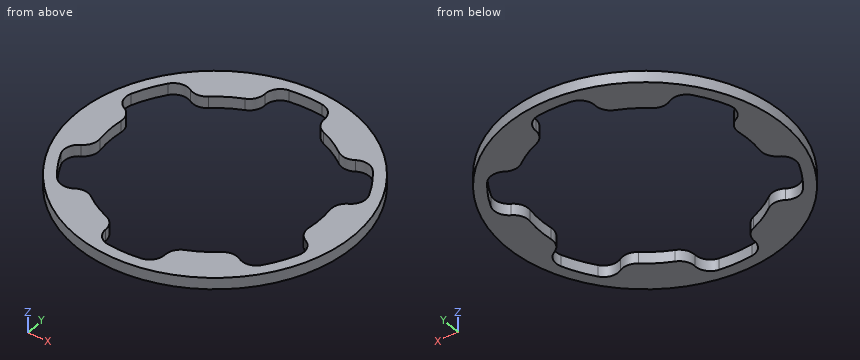
Autodesk Inventor part; units mm, degrees
ref_plane "YZ Plane" through (0, 0, 0) normal (1, 0, 0) x (0, 1, 0)
ref_plane "XZ Plane" through (0, 0, 0) normal (0, 1, 0) x (-1, 0, 0)
ref_plane "XY Plane" through (0, 0, 0) normal (0, 0, 1) x (1, 0, 0)
sketch "MAXSpline Spacer Profile" plane through (0, 0, 0) normal (0, 0, 1) x (1, 0, 0)
  circle A0 centre (0, 0) radius 19.05
  arc A1 (15.22, 4.1356) -> (16.1399, 6.7328) centre (14.2452, 5.9424) ccw
  arc A2 (15.22, 4.1356) -> (14.1626, 2.0366) centre (16.1947, 2.3288) ccw
  arc A3 (14.1626, -2.0366) -> (14.1626, 2.0366) centre (0, 0) ccw
  arc A4 (14.1626, -2.0366) -> (15.22, -4.1356) centre (16.1947, -2.3288) ccw
  arc A5 (16.1399, -6.7328) -> (15.22, -4.1356) centre (14.2452, -5.9424) ccw
  arc A6 (13.9007, -10.6112) -> (16.1399, -6.7328) centre (0, 0) ccw
  arc A7 (11.1915, -11.1131) -> (13.9007, -10.6112) centre (12.2689, -9.3655) ccw
  arc A8 (11.1915, -11.1131) -> (8.845, -11.2469) centre (10.1141, -12.8607) ccw
  arc A9 (5.3176, -13.2835) -> (8.845, -11.2469) centre (0, 0) ccw
  arc A10 (5.3176, -13.2835) -> (4.0285, -15.2487) centre (6.0806, -15.1894) ccw
  arc A11 (2.2392, -17.344) -> (4.0285, -15.2487) centre (1.9763, -15.3079) ccw
  arc A12 (-2.2392, -17.344) -> (2.2392, -17.344) centre (0, 0) ccw
  arc A13 (-4.0285, -15.2487) -> (-2.2392, -17.344) centre (-1.9763, -15.3079) ccw
  arc A14 (-4.0285, -15.2487) -> (-5.3176, -13.2835) centre (-6.0806, -15.1894) ccw
  arc A15 (-8.845, -11.2469) -> (-5.3176, -13.2835) centre (0, 0) ccw
  arc A16 (-8.845, -11.2469) -> (-11.1915, -11.1131) centre (-10.1141, -12.8607) ccw
  arc A17 (-13.9007, -10.6112) -> (-11.1915, -11.1131) centre (-12.2689, -9.3655) ccw
  arc A18 (-16.1399, -6.7328) -> (-13.9007, -10.6112) centre (0, 0) ccw
  arc A19 (-15.22, -4.1356) -> (-16.1399, -6.7328) centre (-14.2452, -5.9424) ccw
  arc A20 (-15.22, -4.1356) -> (-14.1626, -2.0366) centre (-16.1947, -2.3288) ccw
  arc A21 (-14.1626, 2.0366) -> (-14.1626, -2.0366) centre (0, 0) ccw
  arc A22 (-14.1626, 2.0366) -> (-15.22, 4.1356) centre (-16.1947, 2.3288) ccw
  arc A23 (-16.1399, 6.7328) -> (-15.22, 4.1356) centre (-14.2452, 5.9424) ccw
  arc A24 (-13.9007, 10.6112) -> (-16.1399, 6.7328) centre (0, 0) ccw
  arc A25 (-11.1915, 11.1131) -> (-13.9007, 10.6112) centre (-12.2689, 9.3655) ccw
  arc A26 (-11.1915, 11.1131) -> (-8.845, 11.2469) centre (-10.1141, 12.8607) ccw
  arc A27 (-5.3176, 13.2835) -> (-8.845, 11.2469) centre (0, 0) ccw
  arc A28 (-5.3176, 13.2835) -> (-4.0285, 15.2487) centre (-6.0806, 15.1894) ccw
  arc A29 (-2.2392, 17.344) -> (-4.0285, 15.2487) centre (-1.9763, 15.3079) ccw
  arc A30 (2.2392, 17.344) -> (-2.2392, 17.344) centre (0, 0) ccw
  arc A31 (4.0285, 15.2487) -> (2.2392, 17.344) centre (1.9763, 15.3079) ccw
  arc A32 (4.0285, 15.2487) -> (5.3176, 13.2835) centre (6.0806, 15.1894) ccw
  arc A33 (8.845, 11.2469) -> (5.3176, 13.2835) centre (0, 0) ccw
  arc A34 (8.845, 11.2469) -> (11.1915, 11.1131) centre (10.1141, 12.8607) ccw
  arc A35 (13.9007, 10.6112) -> (11.1915, 11.1131) centre (12.2689, 9.3655) ccw
  arc A36 (16.1399, 6.7328) -> (13.9007, 10.6112) centre (0, 0) ccw
  arc A37 (17.4067, -2.0716) -> (17.4067, 2.0716) centre (0, 0) ccw
  arc A38 (15.7454, -1.8738) -> (17.4067, -2.0716) centre (16.5761, -1.9727) ccw
  arc A39 (15.7454, -1.8738) -> (15.7454, 1.8738) centre (0, 0) ccw
  arc A40 (17.4067, 2.0716) -> (15.7454, 1.8738) centre (16.5761, 1.9727) ccw
  arc A41 (10.4974, 14.0389) -> (6.9093, 16.1104) centre (0, 0) ccw
  arc A42 (9.4955, 12.699) -> (10.4974, 14.0389) centre (9.9964, 13.3689) ccw
  arc A43 (9.4955, 12.699) -> (6.2499, 14.5728) centre (0, 0) ccw
  arc A44 (6.9093, 16.1104) -> (6.2499, 14.5728) centre (6.5796, 15.3416) ccw
  arc A45 (-6.9093, 16.1104) -> (-10.4974, 14.0389) centre (0, 0) ccw
  arc A46 (-6.2499, 14.5728) -> (-6.9093, 16.1104) centre (-6.5796, 15.3416) ccw
  arc A47 (-6.2499, 14.5728) -> (-9.4955, 12.699) centre (0, 0) ccw
  arc A48 (-10.4974, 14.0389) -> (-9.4955, 12.699) centre (-9.9964, 13.3689) ccw
  arc A49 (-17.4067, 2.0716) -> (-17.4067, -2.0716) centre (0, 0) ccw
  arc A50 (-15.7454, 1.8738) -> (-17.4067, 2.0716) centre (-16.5761, 1.9727) ccw
  arc A51 (-15.7454, 1.8738) -> (-15.7454, -1.8738) centre (0, 0) ccw
  arc A52 (-17.4067, -2.0716) -> (-15.7454, -1.8738) centre (-16.5761, -1.9727) ccw
  arc A53 (-10.4974, -14.0389) -> (-6.9093, -16.1104) centre (0, 0) ccw
  arc A54 (-9.4955, -12.699) -> (-10.4974, -14.0389) centre (-9.9964, -13.3689) ccw
  arc A55 (-9.4955, -12.699) -> (-6.2499, -14.5728) centre (0, 0) ccw
  arc A56 (-6.9093, -16.1104) -> (-6.2499, -14.5728) centre (-6.5796, -15.3416) ccw
  arc A57 (6.9093, -16.1104) -> (10.4974, -14.0389) centre (0, 0) ccw
  arc A58 (6.2499, -14.5728) -> (6.9093, -16.1104) centre (6.5796, -15.3416) ccw
  arc A59 (6.2499, -14.5728) -> (9.4955, -12.699) centre (0, 0) ccw
  arc A60 (10.4974, -14.0389) -> (9.4955, -12.699) centre (9.9964, -13.3689) ccw
  dimension "d0" = 38.1
sketch "Sketch1" plane through (0, 0, 0) normal (0, 0, 1) x (1, 0, 0)
  circle A0 centre (0, 0) radius 19.05
  arc A1 (15.22, 4.1356) -> (16.1399, 6.7328) centre (14.2452, 5.9424) ccw
  arc A2 (15.22, 4.1356) -> (14.1626, 2.0366) centre (16.1947, 2.3288) ccw
  arc A3 (14.1626, -2.0366) -> (14.1626, 2.0366) centre (0, 0) ccw
  arc A4 (14.1626, -2.0366) -> (15.22, -4.1356) centre (16.1947, -2.3288) ccw
  arc A5 (16.1399, -6.7328) -> (15.22, -4.1356) centre (14.2452, -5.9424) ccw
  arc A6 (13.9007, -10.6112) -> (16.1399, -6.7328) centre (0, 0) ccw
  arc A7 (11.1915, -11.1131) -> (13.9007, -10.6112) centre (12.2689, -9.3655) ccw
  arc A8 (11.1915, -11.1131) -> (8.845, -11.2469) centre (10.1141, -12.8607) ccw
  arc A9 (5.3176, -13.2835) -> (8.845, -11.2469) centre (0, 0) ccw
  arc A10 (5.3176, -13.2835) -> (4.0285, -15.2487) centre (6.0806, -15.1894) ccw
  arc A11 (2.2392, -17.344) -> (4.0285, -15.2487) centre (1.9763, -15.3079) ccw
  arc A12 (-2.2392, -17.344) -> (2.2392, -17.344) centre (0, 0) ccw
  arc A13 (-4.0285, -15.2487) -> (-2.2392, -17.344) centre (-1.9763, -15.3079) ccw
  arc A14 (-4.0285, -15.2487) -> (-5.3176, -13.2835) centre (-6.0806, -15.1894) ccw
  arc A15 (-8.845, -11.2469) -> (-5.3176, -13.2835) centre (0, 0) ccw
  arc A16 (-8.845, -11.2469) -> (-11.1915, -11.1131) centre (-10.1141, -12.8607) ccw
  arc A17 (-13.9007, -10.6112) -> (-11.1915, -11.1131) centre (-12.2689, -9.3655) ccw
  arc A18 (-16.1399, -6.7328) -> (-13.9007, -10.6112) centre (0, 0) ccw
  arc A19 (-15.22, -4.1356) -> (-16.1399, -6.7328) centre (-14.2452, -5.9424) ccw
  arc A20 (-15.22, -4.1356) -> (-14.1626, -2.0366) centre (-16.1947, -2.3288) ccw
  arc A21 (-14.1626, 2.0366) -> (-14.1626, -2.0366) centre (0, 0) ccw
  arc A22 (-14.1626, 2.0366) -> (-15.22, 4.1356) centre (-16.1947, 2.3288) ccw
  arc A23 (-16.1399, 6.7328) -> (-15.22, 4.1356) centre (-14.2452, 5.9424) ccw
  arc A24 (-13.9007, 10.6112) -> (-16.1399, 6.7328) centre (0, 0) ccw
  arc A25 (-11.1915, 11.1131) -> (-13.9007, 10.6112) centre (-12.2689, 9.3655) ccw
  arc A26 (-11.1915, 11.1131) -> (-8.845, 11.2469) centre (-10.1141, 12.8607) ccw
  arc A27 (-5.3176, 13.2835) -> (-8.845, 11.2469) centre (0, 0) ccw
  arc A28 (-5.3176, 13.2835) -> (-4.0285, 15.2487) centre (-6.0806, 15.1894) ccw
  arc A29 (-2.2392, 17.344) -> (-4.0285, 15.2487) centre (-1.9763, 15.3079) ccw
  arc A30 (2.2392, 17.344) -> (-2.2392, 17.344) centre (0, 0) ccw
  arc A31 (4.0285, 15.2487) -> (2.2392, 17.344) centre (1.9763, 15.3079) ccw
  arc A32 (4.0285, 15.2487) -> (5.3176, 13.2835) centre (6.0806, 15.1894) ccw
  arc A33 (8.845, 11.2469) -> (5.3176, 13.2835) centre (0, 0) ccw
  arc A34 (8.845, 11.2469) -> (11.1915, 11.1131) centre (10.1141, 12.8607) ccw
  arc A35 (13.9007, 10.6112) -> (11.1915, 11.1131) centre (12.2689, 9.3655) ccw
  arc A36 (16.1399, 6.7328) -> (13.9007, 10.6112) centre (0, 0) ccw
  arc A37 (17.4067, -2.0716) -> (17.4067, 2.0716) centre (0, 0) ccw
  arc A38 (15.7454, -1.8738) -> (17.4067, -2.0716) centre (16.5761, -1.9727) ccw
  arc A39 (15.7454, -1.8738) -> (15.7454, 1.8738) centre (0, 0) ccw
  arc A40 (17.4067, 2.0716) -> (15.7454, 1.8738) centre (16.5761, 1.9727) ccw
  arc A41 (10.4974, 14.0389) -> (6.9093, 16.1104) centre (0, 0) ccw
  arc A42 (9.4955, 12.699) -> (10.4974, 14.0389) centre (9.9964, 13.3689) ccw
  arc A43 (9.4955, 12.699) -> (6.2499, 14.5728) centre (0, 0) ccw
  arc A44 (6.9093, 16.1104) -> (6.2499, 14.5728) centre (6.5796, 15.3416) ccw
  arc A45 (-6.9093, 16.1104) -> (-10.4974, 14.0389) centre (0, 0) ccw
  arc A46 (-6.2499, 14.5728) -> (-6.9093, 16.1104) centre (-6.5796, 15.3416) ccw
  arc A47 (-6.2499, 14.5728) -> (-9.4955, 12.699) centre (0, 0) ccw
  arc A48 (-10.4974, 14.0389) -> (-9.4955, 12.699) centre (-9.9964, 13.3689) ccw
  arc A49 (-17.4067, 2.0716) -> (-17.4067, -2.0716) centre (0, 0) ccw
  arc A50 (-15.7454, 1.8738) -> (-17.4067, 2.0716) centre (-16.5761, 1.9727) ccw
  arc A51 (-15.7454, 1.8738) -> (-15.7454, -1.8738) centre (0, 0) ccw
  arc A52 (-17.4067, -2.0716) -> (-15.7454, -1.8738) centre (-16.5761, -1.9727) ccw
  arc A53 (-10.4974, -14.0389) -> (-6.9093, -16.1104) centre (0, 0) ccw
  arc A54 (-9.4955, -12.699) -> (-10.4974, -14.0389) centre (-9.9964, -13.3689) ccw
  arc A55 (-9.4955, -12.699) -> (-6.2499, -14.5728) centre (0, 0) ccw
  arc A56 (-6.9093, -16.1104) -> (-6.2499, -14.5728) centre (-6.5796, -15.3416) ccw
  arc A57 (6.9093, -16.1104) -> (10.4974, -14.0389) centre (0, 0) ccw
  arc A58 (6.2499, -14.5728) -> (6.9093, -16.1104) centre (6.5796, -15.3416) ccw
  arc A59 (6.2499, -14.5728) -> (9.4955, -12.699) centre (0, 0) ccw
  arc A60 (10.4974, -14.0389) -> (9.4955, -12.699) centre (9.9964, -13.3689) ccw
extrude "Extrusion1" add sketch "Sketch1" along normal mid plane 1.5875 contours A0 | A38 A39 A40 A37 | A42 A43 A44 A41 | A46 A47 A48 A45 | A50 A51 A52 A49 | A54 A55 A56 A53 | A58 A59 A60 A57
extrude "Extrusion2" [suppressed]
fillet "Fillet1" [suppressed]
mirror "Mirror1" [suppressed]
properties part number "MAXSpline Spacers" material "Acetal Resin, Black"
Input: part model. Units: mm. Frame: model coordinates. Coordinates: 2 decimals unless noted, no trailing zeros. Write each loop counter-clockwise with the first axis right and the second up, starting at its lowest first coordinate (ties: lowest second). Pieces come first, ordered by that corner, then holes. Notation, with made-up numbers: M 5.25,-5 L 60.25,-5 A20 cw 60.25,29 Z; hole C 62.5,-25 d8. An arc over 180 degrees is marked long. Answer as a JSON object with one key per item and string values. Group by question number.
(1) Section A-A on x = 0. Output: boundary loops of the cut face in (y, z).
(2) Section B-B on y = 0. Output: boundary loops of the cut face in (x, z).
(3) Ray query, line 1 along Y through (x, z) = (-0.5, 0.4); line 2 along X through (y, z) = (0.5, -0.4); line 3 along Y through (x, z) = (-15.5, -0.5). Return the intervals inside material, ascending. Write a range as [from, to].
Result set:
{
 "1": {"outline": "M -19.05,-0.79 L -17.49,-0.79 L -17.49,0.79 L -19.05,0.79 Z; M 17.49,-0.79 L 19.05,-0.79 L 19.05,0.79 L 17.49,0.79 Z"},
 "2": {"outline": "M -19.05,-0.79 L -14.31,-0.79 L -14.31,0.79 L -19.05,0.79 Z; M 14.31,-0.79 L 19.05,-0.79 L 19.05,0.79 L 14.31,0.79 Z"},
 "3": {"line 1": "y = [-19.04, -17.48], [17.48, 19.04]", "line 2": "x = [-19.04, -14.3], [14.3, 19.04]", "line 3": "y = [-11.07, -8.1], [-4.32, 4.32], [8.1, 11.07]"}
}
